Design review of the part built by this model. Coordinates are the model's own, in mm. A direction names the side the tool comes from. Coordinates: 2 decimals unless noted, no trailing zeros. Order: outer loops, then holes, each group sorted by start corner. A loop starts at its lowest first (then second) coordinate and runs counter-clockwise, first axis right, second up. Notation, with made-up numbers: M 66,80 L 107,80 A14 ccw 107,84 Z; hole C 9.5,20.25 d8. An arc over 180 degrees is marked long. Answer in a Markdown table with one row per item.
from build123d import *

# Parameters (mm, degrees)
ESBO_O1_W                = 107
ESBO_O1_H                = 28
RESSALTO_EXTRUS_O1_DEPTH = 135
CASCA1_T                 = -0.75
PADR_O_LINEAR1_OUTLINE_W = 107
PADR_O_LINEAR1_OUTLINE_H = 109
PADR_O_LINEAR1_DEPTH     = 135
ESBO_O2_W                = 105.5
ESBO_O2_H                = 26.5
CORTE_EXTRUS_O1_DEPTH    = 134.25


# Read off the part's stored shape, not the designer's step: Padrão linear1
with BuildPart() as part:
    # Esboço1 → Ressalto-extrusão1 (new body)
    with BuildSketch(Plane.XY):
        Rectangle(ESBO_O1_W, ESBO_O1_H)
    extrude(amount=RESSALTO_EXTRUS_O1_DEPTH)

    # Casca1
    casca1_openings = [part.faces().sort_by_distance(p)[0] for p in [
        (0, 0, 135),
    ]]
    offset(amount=CASCA1_T, openings=casca1_openings, kind=Kind.INTERSECTION)

    # Padrão linear1 outline → Padrão linear1 (add)
    with BuildSketch(Plane.XY):
        with Locations((0, 68.5)):
            Rectangle(PADR_O_LINEAR1_OUTLINE_W, PADR_O_LINEAR1_OUTLINE_H)
    extrude(amount=PADR_O_LINEAR1_DEPTH)

    # Esboço2 → Corte-extrusão1 (cut)
    with BuildSketch(Plane.XY.offset(135)):
        Rectangle(ESBO_O2_W, ESBO_O2_H)
        with Locations((0, 27.25)):
            Rectangle(ESBO_O2_W, ESBO_O2_H)
        with Locations((0, 54.5)):
            Rectangle(ESBO_O2_W, ESBO_O2_H)
        with Locations((0, 81.75)):
            Rectangle(ESBO_O2_W, ESBO_O2_H)
        with Locations((0, 109)):
            Rectangle(ESBO_O2_W, ESBO_O2_H)
    extrude(amount=-CORTE_EXTRUS_O1_DEPTH, mode=Mode.SUBTRACT)


solid = part.part
(1) Insertion check: pin 1 Ø2 at (x, y) = (-9.5, 81.5) entering from +Z. The pin has a flat end and moves straight along its axis. Give the tip position at first contact, or say it passes through.
Return value:
| item | result |
|---|---|
| pin 1 | stops at z = 0.75 |
(2) Add section B-B, the plane z = 15. Give the boundary of the cut face in (x, y).
Return value:
| item | result |
|---|---|
| outline | M -53.5,-14 L 53.5,-14 L 53.5,123 L -53.5,123 Z; hole M -52.75,-13.25 L 52.75,-13.25 L 52.75,13.25 L -52.75,13.25 Z; hole M -52.75,14 L 52.75,14 L 52.75,40.5 L -52.75,40.5 Z; hole M -52.75,41.25 L 52.75,41.25 L 52.75,67.75 L -52.75,67.75 Z; hole M -52.75,68.5 L 52.75,68.5 L 52.75,95 L -52.75,95 Z; hole M -52.75,95.75 L 52.75,95.75 L 52.75,122.25 L -52.75,122.25 Z |
(3) For line 1 along Y through (x, z) = (36, 30); line 2 along X through (y, z) = (17, 112.5); line 3 along Z through (x, y) = (28, 37.5), list the stretches that pass through material, from the lowest coordinate up. Write a range as from..to.
Return value:
| item | result |
|---|---|
| line 1 | y = -14..-13.25, 13.25..14, 40.5..41.25, 67.75..68.5, 95..95.75, 122.25..123 |
| line 2 | x = -53.5..-52.75, 52.75..53.5 |
| line 3 | z = 0..0.75 |
(4) For faces 1 (the flat face through (-1, -14, 67)), 2 (the flat face through (-52.75, 109, 69)), list the 3-axis set-ups (+Z, -Z, +X, -X, +Y, -Y) from which the entire face can be reached by the end or side of a thin tool; tool diameter is ignored.
Return value:
| item | result |
|---|---|
| face 1 | +Z, -Z, +X, -X, -Y |
| face 2 | +Z |
(5) Draft analysis for pull direction X (two halves, no side actions). For faces 3 (the flat face through (52.75, 109, 69)), 4 (the flat face through (53.5, 54, 67)), 5 (the flat face through (-1, 55, 0)), state which applies: pulls with the +X half, pulls with the -X half, needs draft (parallel to the pull), parting line crosses it, or undercut.
Return value:
| item | result |
|---|---|
| face 3 | undercut |
| face 4 | pulls with the +X half |
| face 5 | needs draft |
(6) Add section A-A, the plane x = -26.5. Give the boundary of the cut face in (y, z), and give its area (3 significant figures).
Return value:
| item | result |
|---|---|
| outline | M -14,0 L 123,0 L 123,135 L 122.25,135 L 122.25,0.75 L 95.75,0.75 L 95.75,135 L 95,135 L 95,0.75 L 68.5,0.75 L 68.5,135 L 67.75,135 L 67.75,0.75 L 41.25,0.75 L 41.25,135 L 40.5,135 L 40.5,0.75 L 14,0.75 L 14,135 L 13.25,135 L 13.25,0.75 L -13.25,0.75 L -13.25,135 L -14,135 Z |
| area | 707 mm2 |
(7) Add section C-C, the plane y = 50. Give the boundary of the cut face in (x, z), and give its area (3 significant figures).
Return value:
| item | result |
|---|---|
| outline | M -53.5,0 L 53.5,0 L 53.5,135 L 52.75,135 L 52.75,0.75 L -52.75,0.75 L -52.75,135 L -53.5,135 Z |
| area | 282 mm2 |
